Work out the finished part from the listing and answer in its coordinate system (mm). Face numbers are marked on the shaded views. Coordinates: 2 decimals unless noted, no trailing zeros. Write each loop counter-clockwise with the first axis right and the second up, starting at its lowest first coordinate (ties: lowest second). Pieces come first, ordered by that corner, then holes. Notation, with made-up numbers: (-5.5, 11.25) - (39.5, 11.25) arc R7 ccw to (39.5, 20.25) - close; hole circle Ø4 at (-32.5, -39). An arc over 180 degrees is marked (long way). One line per item, written item: value.
Autodesk Inventor part; units mm, degrees
ref_plane "YZ Plane" through (0, 0, 0) normal (1, 0, 0) x (0, 1, 0)
ref_plane "XZ Plane" through (0, 0, 0) normal (0, 1, 0) x (-1, 0, 0)
ref_plane "XY Plane" through (0, 0, 0) normal (0, 0, 1) x (1, 0, 0)
sketch "Sketch1" plane through (0, 0, 0) normal (0, 1, 0) x (-1, 0, 0)
  line L0 (9.5, 25) -> (-9.5, 25)
  line L1 (-9.5, 25) -> (-9.5, -25)
  line L2 (-9.5, -25) -> (9.5, -25)
  line L3 (9.5, -25) -> (9.5, 25)
  line L4 (9.5, 25) -> (-9.5, -25) construction
  line L5 (-9.5, 25) -> (9.5, -25) construction
  circle A0 centre (-4.5, -18) radius 2.6
  circle A1 centre (-4.5, 18) radius 2.6
  point P0 (0, 0)
  dimension "d0" = 50
  dimension "d1" = 19
  dimension "d2" = 5.2
  dimension "d3" = 5.2
  dimension "d4" = 36
  dimension "d5" = 5
  dimension "d6" = 18
extrude "Extrusion1" add sketch "Sketch1" along normal blind 6
properties part number "Fuhrungschiene(n)"
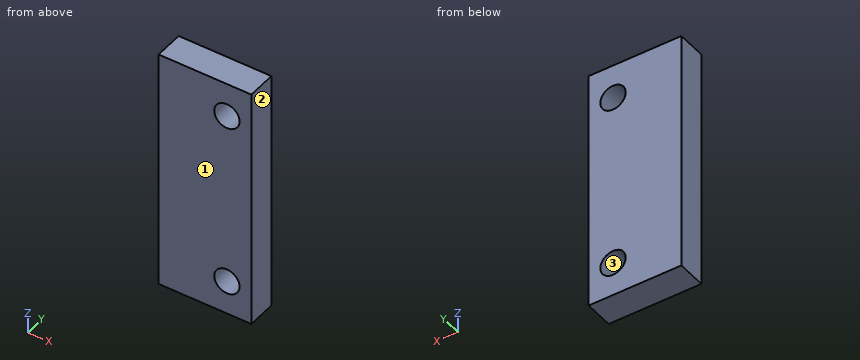
Item 1: Given pin 1 (4 mm diameter, centred on x = 4.5, z = 18, fed in from -Y), flat-ended and moving along its own axis, determine where the tip first touches the part or whether it passes through.
Evaluation:
pin 1: passes through
Item 2: Consider probe 1 along Z at (x, y) = (4.5, 3.05); probe 2 along X at (y, z) = (2.65, -20); probe 3 along X at (y, z) = (1.9, 19.5). Determine where each line is inside the solid, lowest interval first.
Evaluation:
probe 1: z = -25 to -20.6, -15.4 to 15.4, 20.6 to 25
probe 2: x = -9.5 to 2.84, 6.16 to 9.5
probe 3: x = -9.5 to 2.38, 6.62 to 9.5
Item 3: Determine the mould class of the marked faces 1, 2 and 3 for opening direction X: +X half, -X half, draft (parallel to the pull), parting line (faces both ways), or undercut.
Evaluation:
face 1: draft
face 2: +X half
face 3: undercut
Item 4: Section A-A, the plane x = 4.5 is taken. Determine the outline of the cut face in (y, z), then the cut area to 3 significant figures.
Evaluation:
outline: (0, -25) - (6, -25) - (6, -20.6) - (0, -20.6) - close; (0, -15.4) - (6, -15.4) - (6, 15.4) - (0, 15.4) - close; (0, 20.6) - (6, 20.6) - (6, 25) - (0, 25) - close
area: 238 mm2
Item 5: Section B-B, the plane z = -18 is taken. Determine the outline of the cut face in (x, y).
Evaluation:
outline: (-9.5, 0) - (1.9, 0) - (1.9, 6) - (-9.5, 6) - close; (7.1, 0) - (9.5, 0) - (9.5, 6) - (7.1, 6) - close
Item 6: Section C-C, the plane y = 1.4 is taken. Determine the outline of the cut face in (x, z).
Evaluation:
outline: (-9.5, -25) - (9.5, -25) - (9.5, 25) - (-9.5, 25) - close; hole circle Ø5.2 at (4.5, -18); hole circle Ø5.2 at (4.5, 18)
